from build123d import *

# Parameters (mm, degrees)
SKETCH1_R           = 0.5
BOSS_EXTRUDE1_DEPTH = 1.4
SKETCH2_R           = 2.35
CUT_EXTRUDE1_DEPTH  = 1
SKETCH3_R           = 3.5
SKETCH3_R_2         = 2.45
BOSS_EXTRUDE2_DEPTH = 2.5
SKETCH4_R           = 1.2
CUT_EXTRUDE2_DEPTH  = 2.4
SKETCH5_R           = 2.45
SKETCH5_R_2         = 1.2
BOSS_EXTRUDE3_DEPTH = 0.1
SKETCH6_W           = 35.735260114
SKETCH6_H           = 17.672039004
CUT_EXTRUDE4_DEPTH  = 4.9


with BuildPart() as part:
    # Sketch1 → Boss-Extrude1 (new body)
    with BuildSketch(Plane(origin=(0, 0, 0), x_dir=(1, 0, 0), z_dir=(0, 1, 0))):
        with BuildLine():
            Line((-15.2, 2), (-2, 2.95))
            Line((-2, 2.95), (-2, 6.35))
            ThreePointArc((-2, 6.35), (0, 8.35), (2, 6.35))
            Line((2, 6.35), (2, 3.5))
            Line((2, 3.5), (15.2, 2))
            ThreePointArc((15.2, 2), (17.2, 0), (15.2, -2))
            Line((15.2, -2), (2, -3.5))
            Line((2, -3.5), (2, -6.35))
            ThreePointArc((2, -6.35), (0, -8.35), (-2, -6.35))
            Line((-2, -6.35), (-2, -2.95))
            Line((-2, -2.95), (-15.2, -2))
            ThreePointArc((-15.2, -2), (-17.2, 0), (-15.2, 2))
        make_face()
        with Locations((0, 6.35)):
            Circle(SKETCH1_R, mode=Mode.SUBTRACT)
        with Locations((0, 4.55)):
            Circle(SKETCH1_R, mode=Mode.SUBTRACT)
        with Locations((0, -4.55)):
            Circle(SKETCH1_R, mode=Mode.SUBTRACT)
        with Locations((0, -6.35)):
            Circle(SKETCH1_R, mode=Mode.SUBTRACT)
        with Locations((-15.2, 0)):
            Circle(SKETCH1_R, mode=Mode.SUBTRACT)
        with Locations((15.2, 0)):
            Circle(SKETCH1_R, mode=Mode.SUBTRACT)
        with Locations((-13.4, 0)):
            Circle(SKETCH1_R, mode=Mode.SUBTRACT)
        with Locations((-11.6, 0)):
            Circle(SKETCH1_R, mode=Mode.SUBTRACT)
        with Locations((-9.8, 0)):
            Circle(SKETCH1_R, mode=Mode.SUBTRACT)
        with Locations((-8, 0)):
            Circle(SKETCH1_R, mode=Mode.SUBTRACT)
        with Locations((-6.2, 0)):
            Circle(SKETCH1_R, mode=Mode.SUBTRACT)
        with Locations((-4.4, 0)):
            Circle(SKETCH1_R, mode=Mode.SUBTRACT)
        with Locations((13.4, 0)):
            Circle(SKETCH1_R, mode=Mode.SUBTRACT)
        with Locations((11.6, 0)):
            Circle(SKETCH1_R, mode=Mode.SUBTRACT)
        with Locations((9.8, 0)):
            Circle(SKETCH1_R, mode=Mode.SUBTRACT)
        with Locations((8, 0)):
            Circle(SKETCH1_R, mode=Mode.SUBTRACT)
        with Locations((6.2, 0)):
            Circle(SKETCH1_R, mode=Mode.SUBTRACT)
        with Locations((4.4, 0)):
            Circle(SKETCH1_R, mode=Mode.SUBTRACT)
    extrude(amount=BOSS_EXTRUDE1_DEPTH)

    # Sketch2 → Cut-Extrude1 (cut)
    with BuildSketch(Plane.XZ):
        Circle(SKETCH2_R)
    extrude(amount=-CUT_EXTRUDE1_DEPTH, mode=Mode.SUBTRACT)

    # Sketch3 → Boss-Extrude2 (add)
    with BuildSketch(Plane(origin=(0, 1.4, 0), x_dir=(1, 0, 0), z_dir=(0, 1, 0))):
        Circle(SKETCH3_R)
        Circle(SKETCH3_R_2, mode=Mode.SUBTRACT)
    extrude(amount=BOSS_EXTRUDE2_DEPTH)

    # Sketch4 → Cut-Extrude2 (cut, through all)
    with BuildSketch(Plane(origin=(0, 1.4, 0), x_dir=(1, 0, 0), z_dir=(0, 1, 0))):
        Circle(SKETCH4_R)
    extrude(amount=-CUT_EXTRUDE2_DEPTH, mode=Mode.SUBTRACT)

    # Sketch5 → Boss-Extrude3 (add)
    with BuildSketch(Plane(origin=(0, 1.4, 0), x_dir=(1, 0, 0), z_dir=(0, 1, 0))):
        Circle(SKETCH5_R)
        Circle(SKETCH5_R_2, mode=Mode.SUBTRACT)
    extrude(amount=BOSS_EXTRUDE3_DEPTH)

    # Sketch6 → Cut-Extrude4 (cut, through all)
    with BuildSketch(Plane.XZ):
        Rectangle(SKETCH6_W, SKETCH6_H)
        with BuildLine():
            Line((-1.868584713, -2.959457918), (-15.2, -2))
            ThreePointArc((-15.2, -2), (-17.2, 0), (-15.2, 2))
            Line((-15.2, 2), (-1.868584713, 2.959457918))
            ThreePointArc((-1.868584713, 2.959457918), (0, 3.5), (1.868584713, 2.959457918))
            Line((1.868584713, 2.959457918), (15.2, 2))
            ThreePointArc((15.2, 2), (17.2, 0), (15.2, -2))
            Line((15.2, -2), (1.868584713, -2.959457918))
            ThreePointArc((1.868584713, -2.959457918), (0, -3.5), (-1.868584713, -2.959457918))
        make_face(mode=Mode.SUBTRACT)
    extrude(amount=-CUT_EXTRUDE4_DEPTH, mode=Mode.SUBTRACT)


solid = part.part
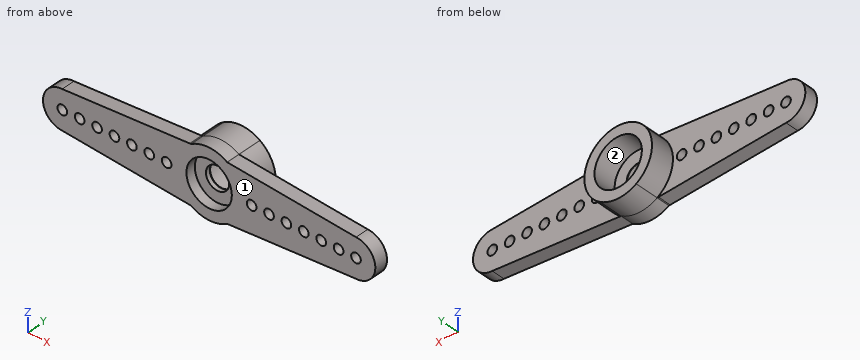
Verification items for the finished model (mm, model axes). Face numbers are marked on the shaded views. Give positions to 0.01 mm unless a question says otherwise; leave off trailing zeros. Loops run counter-clockwise (first coordinate to the right, second up) from the corner with the lowest first, then second, coordinate; pieces in that order, holes last.
1) Depth check by flat-ended pin: pin 1 Ø1.9 at (x, z) = (0, 0) entering from -Y; pin 2 Ø3 at (x, z) = (13, 1) entering from +Y; pin 3 Ø4 at (x, z) = (0, 0) entering from +Y; pin 4 Ø1 at (y, z) = (2, -1.5) entering from +X. Enter the tip coordinate at first touch or a pass-through.
2) Draft check along X on the marked faces 1 and 2. Enter one of: pulls with the +X half, pulls with the -X half, needs draft (parallel to the pull), parting line crosses it, or undercut.
3) Sectioned sample at B-B, the plane y = 2.5. Enter the section's corners in (x, z), then the cut area to 3 significant figures.
4) Sectioned sample at C-C, the plane x = 8. Enter the section's corners in (y, z).
5) Sectioned sample at A-A, the plane x = 13.4. Enter the section's corners in (y, z).
6) Thickness scan on line 1 along X through (y, z) = (2.75, 0); line 2 along Y through (x, z) = (-5, -1); line 3 along X through (y, z) = (0.25, 1.25). Record the ranges inside material, lowest first.
Answers:
1. pin 1: passes through
1. pin 2: stops at y = 1.4
1. pin 3: stops at y = 1.5
1. pin 4: stops at x = 3.35
2. face 1: needs draft
2. face 2: undercut
3. outline: circle Ø7 at (0, 0); hole circle Ø4.9 at (0, 0)
3. area: 19.6 mm2
4. outline: (0, -2.52) - (1.4, -2.52) - (1.4, -0.5) - (0, -0.5) - close; (0, 0.5) - (1.4, 0.5) - (1.4, 2.52) - (0, 2.52) - close
5. outline: (0, -2.13) - (1.4, -2.13) - (1.4, -0.5) - (0, -0.5) - close; (0, 0.5) - (1.4, 0.5) - (1.4, 2.13) - (0, 2.13) - close
6. line 1: x = -3.5 to -2.45, 2.45 to 3.5
6. line 2: y = 0 to 1.4
6. line 3: x = -16.76 to -1.99, 1.99 to 16.76
